from build123d import *

# Parameters (mm, degrees)
BOX012_W          = 68.4
BOX012_H          = 80
BOX012_DEPTH      = 43
CYLINDER003_R     = 1.5
CYLINDER003_DEPTH = 50
ARRAY005_X_COUNT  = 2
ARRAY005_X_PITCH  = 75
ARRAY005_Y_COUNT  = 2
ARRAY005_Y_PITCH  = 31
CYLINDER004_R     = 1.9
CYLINDER004_DEPTH = 10
ARRAY_X_COUNT     = 7
ARRAY_X_PITCH     = 10
ARRAY_Y_COUNT     = 8
ARRAY_Y_PITCH     = 10
BOX010_W          = 80.4
BOX010_H          = 60
BOX010_DEPTH      = 43
CHAMFER001_SIZE   = 25
BOX011_W          = 68.4
BOX011_H          = 80
BOX011_DEPTH      = 40
BOX009_W          = 80.4
BOX009_H          = 80
BOX009_DEPTH      = 46
CHAMFER002_SIZE   = 20


with BuildPart() as v_cube_extract001:
    # Box012 → Box012 (new body)
    with BuildSketch(Plane(origin=(6, 0, 3), x_dir=(1, 0, 0), z_dir=(0, 0, 1))):
        with Locations((34.2, 40)):
            Rectangle(BOX012_W, BOX012_H)
    extrude(amount=BOX012_DEPTH)


with BuildPart() as screw_hole_array:
    # Cylinder003 → Cylinder003 (new body)
    with BuildSketch(Plane.XY.offset(-40)):
        Circle(CYLINDER003_R)
    extrude(amount=CYLINDER003_DEPTH)

    # Array005 X: screw hole array ×2


with BuildPart() as screw_hole_array_1:
    add(screw_hole_array.part)
    with Locations(*[(i * ARRAY005_X_PITCH, 0, 0) for i in range(1, ARRAY005_X_COUNT)]):
        add(screw_hole_array.part)

    # Array005 Y: screw hole array ×2


with BuildPart() as screw_hole_array_2:
    add(screw_hole_array_1.part)
    with Locations(*[(0, i * ARRAY005_Y_PITCH, 0) for i in range(1, ARRAY005_Y_COUNT)]):
        add(screw_hole_array_1.part)


with BuildPart() as screw_hole_array_3:
    # Array005 placement: moved
    add(screw_hole_array_2.part.moved(Location((2.7, 24.5, 43))))


with BuildPart() as attachment_hole_array:
    # Cylinder004 → Cylinder004 (new body)
    with BuildSketch(Plane.XY):
        Circle(CYLINDER004_R)
    extrude(amount=CYLINDER004_DEPTH)

    # Array X: attachment hole array ×7


with BuildPart() as attachment_hole_array_1:
    add(attachment_hole_array.part)
    with Locations(*[(i * ARRAY_X_PITCH, 0, 0) for i in range(1, ARRAY_X_COUNT)]):
        add(attachment_hole_array.part)

    # Array Y: attachment hole array ×8


with BuildPart() as attachment_hole_array_2:
    add(attachment_hole_array_1.part)
    with Locations(*[(0, i * ARRAY_Y_PITCH, 0) for i in range(1, ARRAY_Y_COUNT)]):
        add(attachment_hole_array_1.part)


with BuildPart() as attachment_hole_array_3:
    # Array placement: moved
    add(attachment_hole_array_2.part.moved(Location((10.2, 5, 0))))


with BuildPart() as v_cube_extract_chamfer:
    # Box010 → Box010 (new body)
    with BuildSketch(Plane(origin=(0, 10, 0), x_dir=(1, 0, 0), z_dir=(0, 0, 1))):
        with Locations((40.2, 30)):
            Rectangle(BOX010_W, BOX010_H)
    extrude(amount=BOX010_DEPTH)

    # Chamfer001
    chamfer001_edges = [v_cube_extract_chamfer.edges().sort_by_distance(p)[0] for p in [
        (40.2, 10, 43),
        (40.2, 70, 43),
    ]]
    chamfer(chamfer001_edges, length=CHAMFER001_SIZE)


with BuildPart() as v_extract_union:
    # Box011 → Box011 (new body)
    with BuildSketch(Plane(origin=(6, 0, 3), x_dir=(1, 0, 0), z_dir=(0, 0, 1))):
        with Locations((34.2, 40)):
            Rectangle(BOX011_W, BOX011_H)
    extrude(amount=BOX011_DEPTH)

    # Fusion005: union v cube extract001, screw hole array, attachment hole array, v cube extract chamfer
    add(v_cube_extract001.part)
    add(screw_hole_array_3.part)
    add(attachment_hole_array_3.part)
    add(v_cube_extract_chamfer.part)


with BuildPart() as v_cut:
    # Box009 → Box009 (new body)
    with BuildSketch(Plane.XY):
        with Locations((40.2, 40)):
            Rectangle(BOX009_W, BOX009_H)
    extrude(amount=BOX009_DEPTH)

    # Chamfer002
    chamfer002_edges = [v_cut.edges().sort_by_distance(p)[0] for p in [
        (40.2, 0, 46),
        (40.2, 80, 46),
    ]]
    chamfer(chamfer002_edges, length=CHAMFER002_SIZE)

    # Cut003002: cut v extract union
    add(v_extract_union.part, mode=Mode.SUBTRACT)


solid = v_cut.part
Here's how the part is built. I have some questions about the finished solid (model axes, mm). A direction names the side the tool comes from. Round coordinates to 2 decimals unless told otherwise and drop trailing zeros. Order: outer loops, then holes, each group sorted by start corner. A loop starts at its lowest first (then second) coordinate and runs counter-clockwise, first axis right, second up. Notation, with made-up numbers: (70, 39.25) -> (104, 39.25) arc R21 ccw to (104, 52.25) -> close; hole circle Ø8 at (54.25, -8.5). An arc over 180 degrees is marked (long way). Return JSON: item names as keys, results as strings.
Q1. I need wall thicknesses on line 1 along Y through (x, z) = (70.2, 0.7); line 2 along X through (y, z) = (24, 42); line 3 along X through (y, z) = (75, 13). Which ranges of each line are inside material? Lowest first, please. Write a range as from..to.
Filled sheet:
{"line 1": "y = 0..3.1, 6.9..10, 70..73.1, 76.9..80", "line 2": "x = 0..1.29, 4.11..6, 74.4..76.29, 79.11..80.4", "line 3": "x = 0..6, 74.4..80.4"}
Q2. If we section it at D-D on x = 56: List the corners of the cut face in (y, z) for me.
Filled sheet:
{"outline": "(0, 0) -> (10, 0) -> (10, 3) -> (0, 3) -> close; (70, 0) -> (80, 0) -> (80, 3) -> (70, 3) -> close"}
Q3. If we section it at B-B on y = 13: List the corners of the cut face in (x, z) for me.
Filled sheet:
{"outline": "(0, 21) -> (6, 21) -> (6, 39) -> (0, 39) -> close; (74.4, 21) -> (80.4, 21) -> (80.4, 39) -> (74.4, 39) -> close"}
Q4. If we section it at A-A on z = 6: List the corners of the cut face in (x, y) for me, plus the area to 3 significant figures.
Filled sheet:
{"outline": "(0, 0) -> (6, 0) -> (6, 10) -> (0, 10) -> close; (0, 70) -> (6, 70) -> (6, 80) -> (0, 80) -> close; (74.4, 0) -> (80.4, 0) -> (80.4, 10) -> (74.4, 10) -> close; (74.4, 70) -> (80.4, 70) -> (80.4, 80) -> (74.4, 80) -> close", "area": "240 mm^2"}
Q5. If we mould it in two halves opening along Y, with no side actions, what happens to faces 3 (the cylindrical face through (59.788, 73.145, 1.479)), 4 (the flat face through (3, 40, 46)), 5 (the flat face through (40, 80, 2)), 6 (the flat face through (3, 10, 36))? For each: released by +Y, released by -Y, zero draft, split by the parting line, or undercut.
Filled sheet:
{"face 3": "undercut", "face 4": "zero draft", "face 5": "released by +Y", "face 6": "released by -Y"}
Q6. If we section it at C-C on x = 40.2: List the corners of the cut face in (y, z) for me.
Filled sheet:
{"outline": "(0, 0) -> (3.1, 0) -> (3.1, 3) -> (0, 3) -> close; (6.9, 0) -> (10, 0) -> (10, 3) -> (6.9, 3) -> close; (70, 0) -> (73.1, 0) -> (73.1, 3) -> (70, 3) -> close; (76.9, 0) -> (80, 0) -> (80, 3) -> (76.9, 3) -> close"}
Q7. For pin 1 Ø11 at (x, y) = (51, 5) entering from +Z; pin 2 Ø6.5 at (x, y) = (2.5, 39) entering from -Z, each with a flat end and sliding along its axis, tell me the tip position at first contact or that it passes through.
Filled sheet:
{"pin 1": "stops at z = 3", "pin 2": "stops at z = 43"}
Q8. Which directions (+Z, -Z, +X, -X, +Y, -Y) give clear straight access to the entire face, cutting with the end or side of a thin tool? Please do faces 1 (the cylindrical face through (22.012, 5.571, 1.479)), 2 (the flat face through (77, 40, 43)).
Filled sheet:
{"face 1": "+Z, -Z", "face 2": "-Z, +X, -X"}
